CAD build for the part. Positions are in the model's coordinates, mm. Face numbers are marked on the shaded views. A direction names the side the tool comes from. Round coordinates to 2 decimals unless told otherwise and drop trailing zeros. Order: outer loops, then holes, each group sorted by start corner. A loop starts at its lowest first (then second) coordinate and runs counter-clockwise, first axis right, second up. Notation, with made-up numbers: (22, -26.5) - (78, -26.5) arc R14 ccw to (78, -22.5) - close; hole circle Ø4 at (44, 38). An arc over 180 degrees is marked (long way). Use one line per item in the form item = value. Start each with the question number.
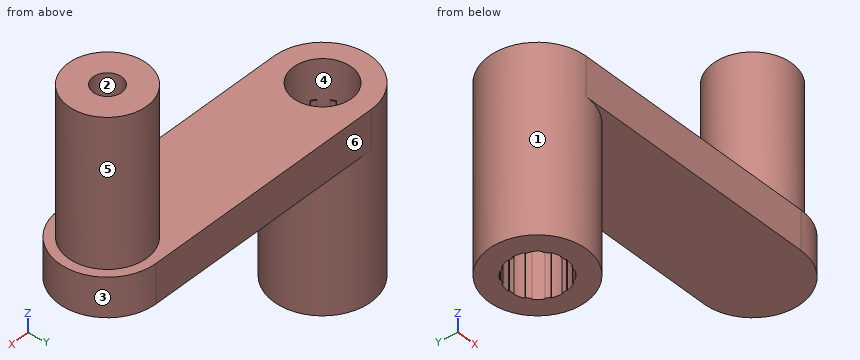
from build123d import *

# Parameters (mm, degrees)
SKETCH005_R        = 2.95
PAD005_DEPTH       = 4
SKETCH007_R        = 4
SKETCH007_R_2      = 1.45
PAD006_DEPTH       = 19
SKETCH016_R        = 4.95
SKETCH016_R_2      = 2.95
PAD015_DEPTH       = 15
SKETCH008_W        = 0.1
SKETCH008_H        = 15
REVOLUTION_ANGLE   = -10
POLARPATTERN_COUNT = 12


with BuildPart() as part:
    # Sketch005 → Pad005 (new body)
    with BuildSketch(Plane.XY.offset(15)):
        with BuildLine():
            ThreePointArc((0, 4.95), (-4.95, 0), (0, -4.95))
            Line((0, -4.95), (25, -4.95))
            ThreePointArc((25, -4.95), (29.95, 0), (25, 4.95))
            Line((25, 4.95), (0, 4.95))
        make_face()
        Circle(SKETCH005_R, mode=Mode.SUBTRACT)
    extrude(amount=PAD005_DEPTH)

    # Sketch007 → Pad006 (join)
    with BuildSketch(Plane.XY.offset(15)):
        with Locations((25, 0)):
            Circle(SKETCH007_R)
        with Locations((25, 0)):
            Circle(SKETCH007_R_2, mode=Mode.SUBTRACT)
    extrude(amount=PAD006_DEPTH)

    # Sketch016 → Pad015 (join)
    with BuildSketch(Plane.XY):
        Circle(SKETCH016_R)
        Circle(SKETCH016_R_2, mode=Mode.SUBTRACT)
    extrude(amount=PAD015_DEPTH)

    # Sketch008 → Revolution (revolve)
    with BuildSketch(Plane.XZ):
        with Locations((2.9, 7.5)):
            Rectangle(SKETCH008_W, SKETCH008_H)
    revolution = revolve(axis=Axis((0, 0, 0), (0, 0, 1)), revolution_arc=REVOLUTION_ANGLE)

    # PolarPattern: Revolution ×12 about axis
    polarpattern_axis = Axis((0, 0, 0), (0, 0, 1))
    for i in range(1, POLARPATTERN_COUNT):
        add(revolution.rotate(polarpattern_axis, i * 360 / POLARPATTERN_COUNT))


solid = part.part
(1) Wall check: line 1 (Y direction, x = 25, z = 29); line 2 (X direction, y = 0, z = 28); line 3 (Z direction, x = 20, y = -2.25). Give the ranges that are in metal, low to high. Write a range as [from, to].
(2) Which spindle directions (+Z, -Z, +X, -X, +Y, -Y) get a long thin tool onto all of the face, cutting with end or side? Do the marked faces 1, 2 and 3. Say none if no direction does.
(3) Slice it at A-A (z = 29). Give the cut face in (x, y), and give its area (3 significant figures).
(4) Slice it at B-B (x = 25.5). Give the cut face in (y, z), and give its area (3 significant figures).
(5) Flat gauge pins, fed straight in: P1, Ø1.4, axis at x = 25, y = 0.5, coming from the +Z side; P2, Ø1, axis at x = 3, z = 13.5, coming from the -Y side; P3, Ø6, axis at x = 16.5, z = 19.5, coming from the -Y side; P4, Ø8, axis at x = 21.5, z = 23.5, coming from the +Y side. Where does each tip first touch, or does it go through?
(6) Slice it at C-C (y = 3.5). Give the cut face in (x, z), and give its area (3 significant figures).
(7) Mould opens along X. For the marked faces 4, 5 and 6 say: pulls with the +X half, pulls with the -X half, needs draft (parallel to the pull), parting line crosses it, or undercut.
Results list:
q1.line_1 = [-4, -1.45], [1.45, 4]
q1.line_2 = [21, 23.55], [26.45, 29]
q1.line_3 = [15, 19]
q2.face_1 = -Z
q2.face_2 = +Z
q2.face_3 = +Z, -Z, +X
q3.outline = circle Ø8 at (25, 0); hole circle Ø2.9 at (25, 0)
q3.area = 43.7 mm²
q4.outline = (-4.92, 15) - (4.92, 15) - (4.92, 19) - (3.97, 19) - (3.97, 34) - (1.36, 34) - (1.36, 19) - (-1.36, 19) - (-1.36, 34) - (-3.97, 34) - (-3.97, 19) - (-4.92, 19) - close
q4.area = 118 mm²
q5.P1 = 19
q5.P2 = -4.27
q5.P3 = -4.95
q5.P4 = 4
q6.outline = (-3.5, 0) - (3.5, 0) - (3.5, 15) - (28.5, 15) - (28.5, 19) - (26.94, 19) - (26.94, 34) - (23.06, 34) - (23.06, 19) - (-3.5, 19) - close
q6.area = 291 mm²
q7.face_4 = undercut
q7.face_5 = parting line crosses it
q7.face_6 = needs draft
